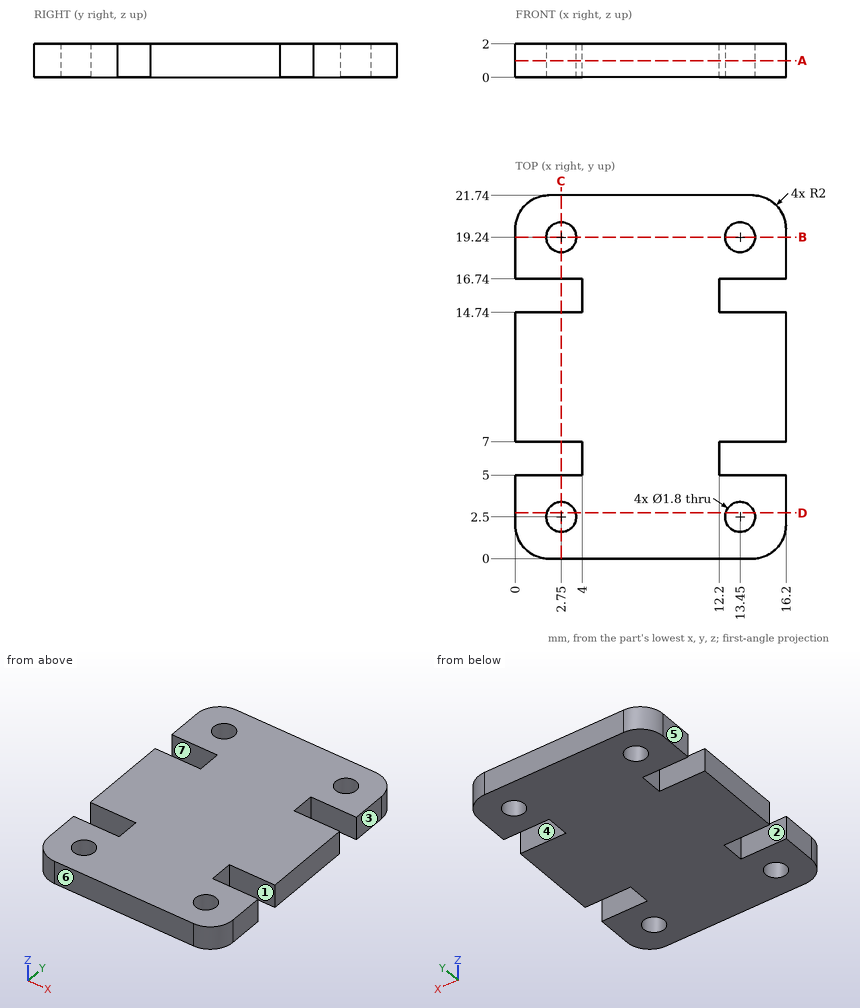
Study the drawing (mm; zero at the part's minimum x, y, z) and answer. A direction names the side the tool comes from. Coordinates: 2 decimals unless noted, no trailing zeros. Order: outer loops, then holes, each group sorted by start corner. A loop starts at its lowest first (then second) coordinate and runs counter-clockwise, first axis right, second up. Notation, with made-up numbers: M 8.5,-2.5 L 37.5,-2.5 A18 cw 37.5,9.5 Z; hole C -7,-37.5 d1. An arc over 180 degrees is marked long. Use CSV: the item, a comma, the result in double quotes.
Q1. Section A-A (z = 1) is taken. Determine the outline of the cut face in (x, y).
Here are the results:
outline,"M 0,2 A2 ccw 2,0 L 14.2,0 A2 ccw 16.2,2 L 16.2,5 L 12.2,5 L 12.2,7 L 16.2,7 L 16.2,14.74 L 12.2,14.74 L 12.2,16.74 L 16.2,16.74 L 16.2,19.74 A2 ccw 14.2,21.74 L 2,21.74 A2 ccw 0,19.74 L 0,16.74 L 4,16.74 L 4,14.74 L 0,14.74 L 0,7 L 4,7 L 4,5 L 0,5 Z; hole C 2.75,2.5 d1.8; hole C 2.75,19.24 d1.8; hole C 13.45,2.5 d1.8; hole C 13.45,19.24 d1.8"
Q2. Section C-C (x = 2.75) is taken. Determine the outline of the cut face in (y, z).
Here are the results:
outline,"M 0,0 L 1.6,0 L 1.6,2 L 0,2 Z; M 3.4,0 L 5,0 L 5,2 L 3.4,2 Z; M 7,0 L 14.74,0 L 14.74,2 L 7,2 Z; M 16.74,0 L 18.34,0 L 18.34,2 L 16.74,2 Z; M 20.14,0 L 21.74,0 L 21.74,2 L 20.14,2 Z"
Q3. Section D-D (y = 2.75) is taken. Determine the outline of the cut face in (x, z), then the cut area to 3 significant figures.
Here are the results:
outline,"M 0,0 L 1.89,0 L 1.89,2 L 0,2 Z; M 3.61,0 L 12.59,0 L 12.59,2 L 3.61,2 Z; M 14.31,0 L 16.2,0 L 16.2,2 L 14.31,2 Z"
area,"25.5 mm2"
Q4. A tool of negligible diameter and unlimited length cuts with its end or side. For the marked faces 1, 2 and 3, from which of +Z, -Z, +X, -X, +Y, -Y can it reach the whole face along a straight path? Write none if from no direction.
Here are the results:
face 1,"+Z, -Z, +X"
face 2,"+Z, -Z, -X"
face 3,"+Z, -Z, +X, +Y, -Y"
Q5. Determine the mould class of the marked faces 4, 5, 6 and 7 for opening direction Y: pulls with the +Y half, pulls with the -Y half, needs draft (parallel to the pull), parting line crosses it, or undercut.
Here are the results:
face 4,"undercut"
face 5,"needs draft"
face 6,"pulls with the -Y half"
face 7,"undercut"
Q6. Straight lines are drawn through the part: L1, parallel to X at y = 2.5, z = 0.75; L2, parallel to Y at x = 13.45, z = 1.4; L3, parallel to Y at x = 3.75, z = 1.55. For each, find the intervals that lie inside material, in ascending order.
Here are the results:
L1,"0 to 1.85, 3.65 to 12.55, 14.35 to 16.2"
L2,"0 to 1.6, 3.4 to 5, 7 to 14.74, 16.74 to 18.34, 20.14 to 21.74"
L3,"0 to 5, 7 to 14.74, 16.74 to 21.74"
Q7. Section B-B (y = 19.24) is taken. Determine the outline of the cut face in (x, z), then the cut area to 3 significant figures.
Here are the results:
outline,"M 0,0 L 1.85,0 L 1.85,2 L 0,2 Z; M 3.65,0 L 12.55,0 L 12.55,2 L 3.65,2 Z; M 14.35,0 L 16.2,0 L 16.2,2 L 14.35,2 Z"
area,"25.2 mm2"
Q8. Given pin 1 Ø1.6 at (x, y) = (2.75, 19.24) entering from +Z; pin 2 Ø1 at (y, z) = (15.5, 1.5) entering from +X; pin 3 Ø0.6 at (y, z) = (5.5, 0.5) entering from -X; pin 4 Ø0.6 at (x, z) = (1.5, 1) entering from -Y, each flat-ended and moving along its own axis, determine where each tip first touches the part or whether it passes through.
Here are the results:
pin 1,"through"
pin 2,"x = 12.2"
pin 3,"x = 4"
pin 4,"y = 0.01"
